```python
from build123d import *
from build123d.topology import SkipClean

# Parameters (mm, degrees)
SKIZZE1_R                         = 3
AUFSATZ_LINEAR_AUSTRAGEN1_DEPTH   = 4
AUFSATZ_LINEAR_AUSTRAGEN1_2_DEPTH = 4
AUFSATZ_LINEAR_START              = 1
SKIZZE2_W                         = 39.730311682
SKIZZE2_H                         = 6
AUFSATZ_LINEAR_AUSTRAGEN2_DEPTH   = 4
SKIZZE3_R                         = 3
AUFSATZ_LINEAR_AUSTRAGEN3_DEPTH   = 34.6252
SCHNITT_LINEAR_AUSTRAGEN1_DEPTH   = 56.942794256
SKIZZE11_W                        = 6
SKIZZE11_H                        = 15
AUFSATZ_LINEAR_AUSTRAGEN8_DEPTH   = 4
SKIZZE12_R                        = 1.7
SCHNITT_LINEAR_AUSTRAGEN6_DEPTH   = 4
SKIZZE14_W                        = 25.08
SKIZZE14_H                        = 6
SCHNITT_LINEAR_AUSTRAGEN8_DEPTH   = 59.228840184
SKIZZE15_W                        = 33.730311682
SKIZZE15_H                        = 5
AUFSATZ_LINEAR_AUSTRAGEN9_DEPTH   = 4
SKIZZE17_R                        = 1.7
SCHNITT_LINEAR_AUSTRAGEN9_DEPTH   = 2
VERRUNDUNG1_R                     = 3


with BuildPart() as part:
    # Skizze1 → Aufsatz-Linear austragen1 (new body)
    with BuildSketch(Plane.XY):
        with Locations((-15.621, 18.161)):
            Circle(SKIZZE1_R)
    extrude(amount=AUFSATZ_LINEAR_AUSTRAGEN1_DEPTH)



with BuildPart() as body_2:
    # Skizze1 → Aufsatz-Linear austragen1 2 (new body)
    with BuildSketch(Plane.XY):
        with Locations(Location((3.459, 18.161, 0), (0, 0, 180))):
            Circle(SKIZZE1_R)
    extrude(amount=AUFSATZ_LINEAR_AUSTRAGEN1_2_DEPTH)


with BuildPart() as part_1:
    add(part.part)

    add(body_2.part)  # Aufsatz-Linear austragen2 merges body 2
    # Skizze2 → Aufsatz-Linear austragen2 (add)
    with BuildSketch(Plane.XY.offset(AUFSATZ_LINEAR_START)):
        with Locations((-9.868250172, 18.161)):
            Rectangle(SKIZZE2_W, SKIZZE2_H)
    extrude(amount=AUFSATZ_LINEAR_AUSTRAGEN2_DEPTH)

    # Skizze3 → Aufsatz-Linear austragen3 (add)
    with BuildSketch(Plane.XY.offset(1)):
        with Locations(Location((-26.733406013, 18.161, 0), (0, 0, 90))):
            Circle(SKIZZE3_R)
        with Locations(Location((6.996905669, 18.161, 0), (0, 0, 90))):
            Circle(SKIZZE3_R)
        with Locations(Location((-26.733406013, 33.161, 0), (0, 0, 180))):
            Circle(SKIZZE3_R)
    extrude(amount=AUFSATZ_LINEAR_AUSTRAGEN3_DEPTH)


with BuildPart() as aufsatz_linear_austragen3_piece_1:
    # of the separate pieces the step leaves, piece 1, a body of its own (aufsatz_linear_austragen3_pieces)
    add(part_1.part.solids().sort_by_distance((-12.621, 18.161, 0))[0])

    # Skizze5 → Schnitt-Linear austragen1 (cut, through all)
    with SkipClean():  # the faces are left unmerged after this step: merging them gives an invalid solid
        with BuildSketch(Plane.XY.offset(5)):
            with BuildLine():
                Line((-26.733406013, 21.161), (-36.757848336, 21.161))
                Line((-36.757848336, 21.161), (-36.757848336, 15.161))
                Line((-36.757848336, 15.161), (-26.733406013, 15.161))
                ThreePointArc((-26.733406013, 15.161), (-29.733406013, 18.161), (-26.733406013, 21.161))
            make_face()
            with BuildLine():
                Line((17.021347992, 15.161), (6.996905669, 15.161))
                ThreePointArc((6.996905669, 15.161), (9.996905669, 18.161), (6.996905669, 21.161))
                Line((6.996905669, 21.161), (17.021347992, 21.161))
                Line((17.021347992, 21.161), (17.021347992, 15.161))
            make_face()
        extrude(amount=-SCHNITT_LINEAR_AUSTRAGEN1_DEPTH, mode=Mode.SUBTRACT)



with BuildPart() as aufsatz_linear_austragen3_piece_2:
    # of the separate pieces the step leaves, piece 2, a body of its own (aufsatz_linear_austragen3_pieces)
    add(part_1.part.solids().sort_by_distance((-29.733406013, 33.161, 1))[0])


with BuildPart() as aufsatz_linear_austragen3_piece_1_1:
    with SkipClean():  # the faces are left unmerged after this step: merging them gives an invalid solid
        add(aufsatz_linear_austragen3_piece_1.part)

        add(aufsatz_linear_austragen3_piece_2.part)  # Aufsatz-Linear austragen8 merges Aufsatz-Linear austragen3 piece 2
        # Skizze11 → Aufsatz-Linear austragen8 (add)
        with BuildSketch(Plane.XY.offset(5)):
            with Locations((-26.733406013, 25.661)):
                Rectangle(SKIZZE11_W, SKIZZE11_H)
        extrude(amount=-AUFSATZ_LINEAR_AUSTRAGEN8_DEPTH)

    # Skizze12 → Schnitt-Linear austragen6 (cut)
    with SkipClean():  # the faces are left unmerged after this step: merging them gives an invalid solid
        with BuildSketch(Plane.XY.offset(35.6252)):
            with Locations((-26.733406013, 33.161)):
                Circle(SKIZZE12_R)
            with Locations(Location((-26.733406013, 18.161, 0), (0, 0, 180))):
                Circle(SKIZZE12_R)
            with Locations(Location((6.996905669, 18.161, 0), (0, 0, 180))):
                Circle(SKIZZE12_R)
        extrude(amount=-SCHNITT_LINEAR_AUSTRAGEN6_DEPTH, mode=Mode.SUBTRACT)

    # Skizze14 → Schnitt-Linear austragen8 (cut, through all)
    with SkipClean():  # the faces are left unmerged after this step: merging them gives an invalid solid
        with BuildSketch(Plane(origin=(0, 0, 1), x_dir=(-1, 0, 0), z_dir=(0, 0, -1))):
            with Locations((6.081, 18.161)):
                Rectangle(SKIZZE14_W, SKIZZE14_H)
        extrude(amount=SCHNITT_LINEAR_AUSTRAGEN8_DEPTH, mode=Mode.SUBTRACT)

    # Skizze15 → Aufsatz-Linear austragen9 (add)
    with BuildSketch(Plane(origin=(0, 0, 1), x_dir=(-1, 0, 0), z_dir=(0, 0, -1))):
        with Locations((6.868250172, 20.661)):
            Rectangle(SKIZZE15_W, SKIZZE15_H)
    extrude(amount=-AUFSATZ_LINEAR_AUSTRAGEN9_DEPTH)

    # Skizze17 → Schnitt-Linear austragen9 (cut)
    with BuildSketch(Plane(origin=(0, 0, 1), x_dir=(-1, 0, 0), z_dir=(0, 0, -1))):
        with Locations((-5.459, 20.161)):
            Circle(SKIZZE17_R)
        with Locations((15.621, 20.161)):
            Circle(SKIZZE17_R)
    extrude(amount=-SCHNITT_LINEAR_AUSTRAGEN9_DEPTH, mode=Mode.SUBTRACT)

    # Verrundung1
    verrundung1_edges = [aufsatz_linear_austragen3_piece_1_1.edges().sort_by_distance(p)[0] for p in [
        (9.996905669, 23.161, 3),
    ]]
    fillet(verrundung1_edges, radius=VERRUNDUNG1_R)


solid = aufsatz_linear_austragen3_piece_1_1.part
```
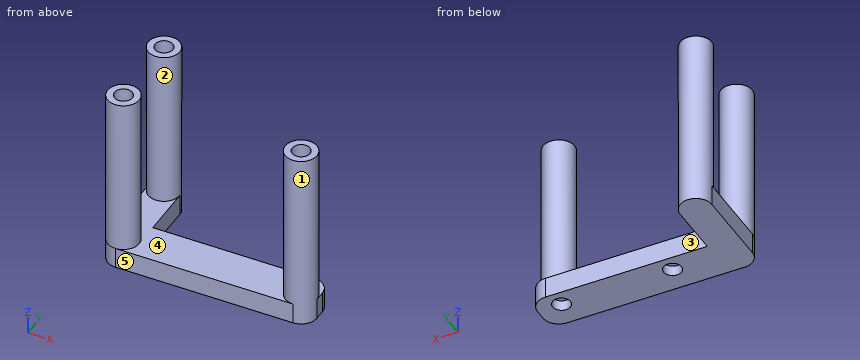
Source: CAD feature listing. Evaluate the final solid. Frame: model axes, mm. Face numbers are marked on the shaded views. A direction names the side the tool comes from. Coordinates: 2 decimals unless noted, no trailing zeros. Loops run counter-clockwise (first coordinate to the right, second up) from the corner with the lowest first, then second, coordinate; pieces in that order, holes last. Notation, with made-up numbers: (76, 36.25) -> (132, 36.25) arc R18 ccw to (132, 69.25) -> close; hole circle Ø4 at (87.25, -7). An arc over 180 degrees is marked (long way). One line per item, written item: value. Start each with the question number.
Q1. Mould query, pull axis X, two halves, no side actions, for the marked faces 1, 2 and 3. Classes: pulls with the +X half, pulls with the -X half, needs draft (parallel to the pull), parting line crosses it, or undercut.
Q2. Section query B-B, the plane y = 34. Return the cut outline in (x, z), and give its area (3 significant figures).
Q3. Set-up query: the marked faces 4 and 5. Return all of +Z, -Z, +X, -X, +Y, -Y with unobstructed straight access to the full face (end or side cutting, diameter ignored); none if empty.
Q4. Section query D-D, the plane y = 27.75. Return the cut outline in (x, z).
Q5. Contact query for flat-ended pins moving along their axis: P1, Ø3, axis at y = 32, z = 12.5, coming from the +X side; P2, Ø12, axis at x = -3, z = 7, coming from the +Y side; P3, Ø4, axis at x = -20.5, y = 25.5, coming from the -Z side; P4, Ø5, axis at y = 22, z = 30.5, coming from the +X side. Output: stop coordinate, or through.
Q6. Section query A-A, the plane z = 27. Return the cut outline in (x, y).
Q7. Section query C-C, the plane x = -7. Return the cut outline in (y, z).
Q8. Line query: line 1 along Y through (x, z) = (-26.5, 29.5); line 2 along X through (y, z) = (17.5, 32); line 3 along X through (y, z) = (20.5, 24). Output: solid intervals per line, ascending.
Results:
1. face 1: undercut
1. face 2: parting line crosses it
1. face 3: needs draft
2. outline: (-29.61, 1) -> (-23.85, 1) -> (-23.85, 35.63) -> (-25.25, 35.63) -> (-25.25, 31.63) -> (-28.21, 31.63) -> (-28.21, 35.63) -> (-29.61, 35.63) -> close
2. area: 188 mm^2
3. face 4: +Z
3. face 5: +Z, -Z, +X, -X, -Y
4. outline: (-29.73, 1) -> (-23.73, 1) -> (-23.73, 5) -> (-29.73, 5) -> close
5. P1: x = -23.73
5. P2: y = 23.16
5. P3: through
5. P4: x = 9.68
6. outline: circle Ø6 at (-26.73, 18.16); circle Ø6 at (-26.73, 33.16); circle Ø6 at (7, 18.16)
7. outline: (15.16, 1) -> (23.16, 1) -> (23.16, 5) -> (15.16, 5) -> close
8. line 1: 15.17 to 21.15, 30.17 to 36.15
8. line 2: -29.66 to -28.3, -25.17 to -23.81, 4.07 to 5.43, 8.56 to 9.92
8. line 3: -28.61 to -24.85, 5.12 to 8.88
